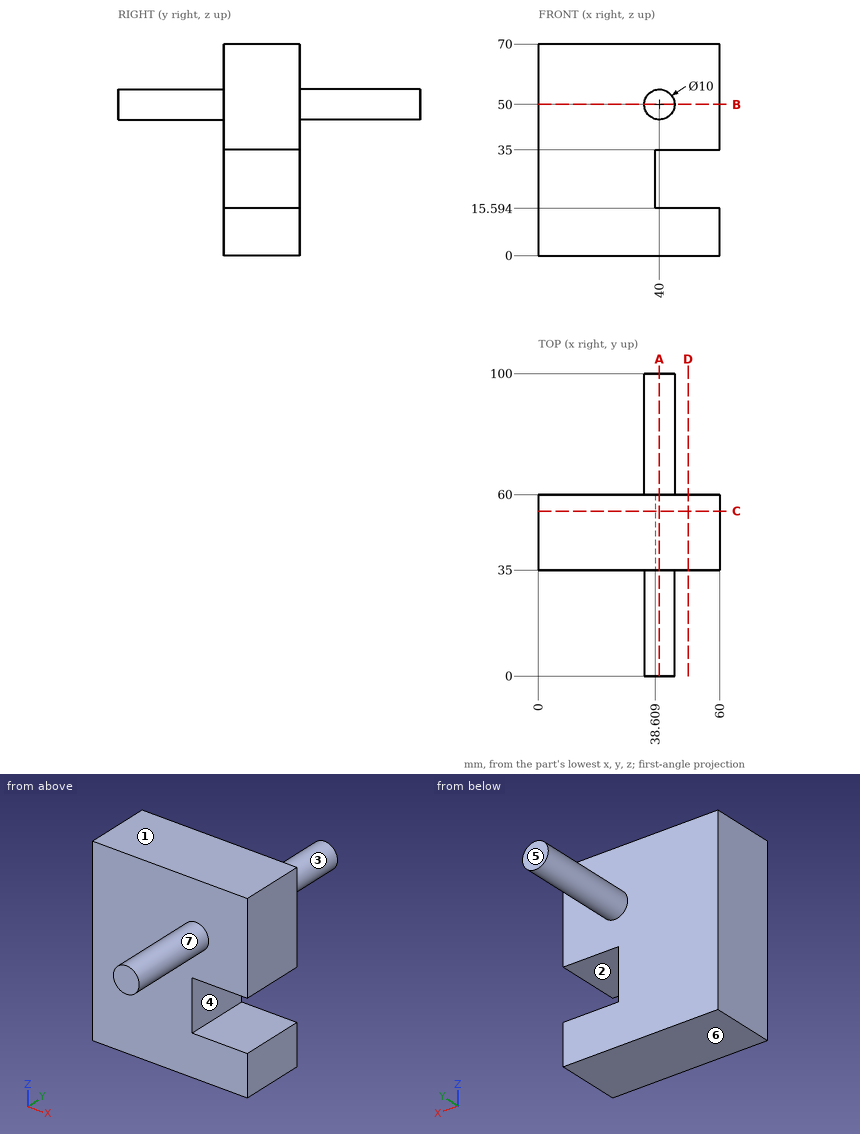
Answer from the drawing. Dimensions are ordinates in mm from the lowest x, y and z of the part. A direction names the side the tool comes from. Coordinates: 2 decimals unless noted, no trailing zeros. Loops run counter-clockwise (first coordinate to the right, second up) from the corner with the lowest first, then second, coordinate; pieces in that order, holes last. Notation, with made-up numbers: (32, -35.75) -> (61, -35.75) arc R35 cw to (61, 2.25) -> close; hole circle Ø1 at (32.25, 78). An arc over 180 degrees is marked (long way). Return JSON: item names as keys, results as strings.
Item 1: Find section B-B (z = 50). Determine the outline of the cut face in (x, y).
Answers:
{"outline": "(0, 35) -> (35, 35) -> (35, 0) -> (45, 0) -> (45, 35) -> (60, 35) -> (60, 60) -> (45, 60) -> (45, 100) -> (35, 100) -> (35, 60) -> (0, 60) -> close"}
Item 2: Find section A-A (x = 40). Determine the outline of the cut face in (y, z).
Answers:
{"outline": "(0, 45) -> (35, 45) -> (35, 35) -> (60, 35) -> (60, 45) -> (100, 45) -> (100, 55) -> (60, 55) -> (60, 70) -> (35, 70) -> (35, 55) -> (0, 55) -> close; (35, 0) -> (60, 0) -> (60, 15.59) -> (35, 15.59) -> close"}
Item 3: For a pull along Z with two mould halves and no side action, classify the marked faces 4, 5, 6 and 7 as +Z half, -Z half, draft (parallel to the pull), parting line (faces both ways), or undercut.
Answers:
{"face 4": "undercut", "face 5": "draft", "face 6": "-Z half", "face 7": "parting line"}
Item 4: Find section D-D (x = 49.5). Determine the outline of the cut face in (y, z), plus the area to 3 significant figures.
Answers:
{"outline": "(35, 0) -> (60, 0) -> (60, 15.59) -> (35, 15.59) -> close; (35, 35) -> (60, 35) -> (60, 70) -> (35, 70) -> close", "area": "1,260 mm2"}
Item 5: Find the intervals of material crossed by probe 1 along Z at (x, y) = (53, 49); probe 2 along X at (y, z) = (51, 17); probe 3 along Y at (x, z) = (20.5, 14), in increasing order.
Answers:
{"probe 1": "z = 0 to 15.59, 35 to 70", "probe 2": "x = 0 to 38.61", "probe 3": "y = 35 to 60"}
Item 6: Flat-ended cylindrical pins translate along their axes: P1, Ø1, axis at x = 8, z = 55.5, coming from the -Y side; P2, Ø6, axis at x = 42.5, y = 74.5, coming from the +Z side; P3, Ø18, axis at x = 27, z = 38, coming from the +Y side. Find the tip coordinate at first contact, or state that the pin passes through.
Answers:
{"P1": "stops at y = 35", "P2": "stops at z = 55", "P3": "stops at y = 60"}
Item 7: Find section C-C (y = 54.5). Determine the outline of the cut face in (x, z), plus the area to 4 significant figures.
Answers:
{"outline": "(0, 0) -> (60, 0) -> (60, 15.59) -> (38.61, 15.59) -> (38.61, 35) -> (60, 35) -> (60, 70) -> (0, 70) -> close", "area": "3,785 mm2"}
Item 8: For the marked faces 1, 2 and 3, determine the directions among +Z, -Z, +X, -X, +Y, -Y from which every point of the face is accessible in a straight line to the end or side of a thin tool.
Answers:
{"face 1": "+Z, +X, -X, +Y, -Y", "face 2": "+X, +Y, -Y", "face 3": "+Y"}
